Build history of the part. All positions in model axes, mm. Face numbers are marked on the shaded views. A direction names the side the tool comes from. Give positions to 0.01 mm unless a question says otherwise; leave off trailing zeros. Order: outer loops, then holes, each group sorted by start corner. A loop starts at its lowest first (then second) coordinate and runs counter-clockwise, first axis right, second up. Notation, with made-up numbers: (83, 56.5) -> (128, 56.5) arc R30 ccw to (128, 92.5) -> close; hole circle Ø9 at (56, 69.25). An arc over 180 degrees is marked (long way). One line per item, written item: value. Start each with the question number.
(1) Saw through at B-B on y = 10. Count the separate pieces of the cut face and the enclosed holes in it, plus the area to 3 significant figures.
(2) Saw through at A-A on z = -18. Give the cut face in (x, y), plus the area to 3 significant figures.
(3) Saw through at C-C on x = 22.5. Give the cut face in (y, z), plus the area to 3 significant figures.
(4) Pin check, flat tips, straight feed: pin 1 (3.5 mm diameter, centred on x = 7.5, z = 6, fed in from +Y); pin 2 (7.5 mm diameter, centred on y = 16, z = 18, fed in from -X); pin 3 (1 mm diameter, centred on x = -40.5, z = -2.5, fed in from +Y). Stop position of each tip, or through.
(5) Which spindle directions (+Z, -Z, +X, -X, +Y, -Y) get a long thin tool onto all of the face, cutting with end or side? Do the marked faces 1, 2 and 3. Say none if no direction does.
(6) Two-plate mould, pull along Y, no slides. Class the marked faces 4, 5, 6 and 7: +Y half, -Y half, draft (parallel to the pull), parting line (faces both ways), or undercut.
(7) Probe line 1 (X direction, y = 21, z = 13.5); line 2 (X direction, y = 11.5, z = 18); line 3 (X direction, y = 6, z = 25.5). List the from-to ranges inside material, lowest first.
Autodesk Inventor part; units mm, degrees
ref_plane "YZ Plane" through (0, 0, 0) normal (1, 0, 0) x (0, 1, 0)
ref_plane "XZ Plane" through (0, 0, 0) normal (0, 1, 0) x (-1, 0, 0)
ref_plane "XY Plane" through (0, 0, 0) normal (0, 0, 1) x (1, 0, 0)
sketch "Sketch1" plane through (0, 0, 0) normal (0, 1, 0) x (-1, 0, 0)
  line L0 (17.7167, 30.9206) -> (-32.2833, 30.9206)
  line L1 (-32.2833, 30.9206) -> (-32.2833, -19.0794)
  line L2 (-32.2833, -19.0794) -> (17.7167, -19.0794)
  line L3 (17.7167, -19.0794) -> (17.7167, 30.9206)
  line L4 (19.7167, 32.9206) -> (-34.2833, 32.9206)
  line L5 (-34.2833, 32.9206) -> (-34.2833, -21.0794)
  line L6 (-34.2833, -21.0794) -> (19.7167, -21.0794)
  line L7 (19.7167, -21.0794) -> (19.7167, 32.9206)
  line L8 (19.7167, 32.9206) -> (54.7167, 32.9206)
  line L9 (54.7167, 32.9206) -> (54.7167, -21.0794)
  line L10 (54.7167, -21.0794) -> (19.7167, -21.0794)
  line L11 (19.7167, -21.0794) -> (19.7167, 32.9206)
  point P0 (0, 0)
  dimension "d0" = 50
  dimension "d1" = 50
  dimension "d2" = 2
  dimension "d3" = 2
  dimension "d4" = 2
  dimension "d5" = 2
  dimension "d6" = 35
  dimension "d7" = 54
extrude "Extrusion1" add sketch "Sketch1" along normal blind 27 contours L7 L6 L5 L4
sketch "Sketch2" plane through (34.2833, 0, 32.9206) normal (1, 0, 0) x (0, 0, -1)
  line L0 (0, 0) -> (0, 27)
  line L1 (54, 0) -> (54, 27)
  line L2 (0, 0) -> (54, 0)
  line L3 (54, 0) -> (54, 2)
  line L4 (54, 2) -> (0, 2)
  line L5 (0, 2) -> (0, 0)
  point P0 (32.9206, 0)
  dimension "d10" = 2
extrude "Extrusion2" add sketch "Sketch2" against normal blind 89
fillet "Fillet1" radius 2 7 edges at (34.2833, 13.5, 32.9206) (34.2833, 13.5, -21.0794) (-19.7167, 14.5, -21.0794) (-19.7167, 14.5, 32.9206) (34.2833, 0, 5.9206) (-10.2167, 0, 32.9206) (-10.2167, 0, -21.0794)
sketch "Sketch3" plane through (-17.7167, 2, 30.9206) normal (0, 1, 0) x (1, 0, 0)
  line L0 (9, 9) -> (1, 9)
  line L1 (1, 9) -> (1, 17)
  line L2 (1, 17) -> (9, 17)
  line L3 (9, 17) -> (9, 9)
  line L4 (50, 0) -> (0, 0)
  line L5 (0, 0) -> (0, 50)
  line L6 (8.05, 9.95) -> (1.95, 9.95)
  line L7 (1.95, 9.95) -> (1.95, 16.05)
  line L8 (1.95, 16.05) -> (8.05, 16.05)
  line L9 (8.05, 16.05) -> (8.05, 9.95)
  line L10 (0, 25) -> (50, 25)
  line L11 (0, 50) -> (50, 50)
  line L12 (50, 50) -> (50, 0)
  line L13 (9, 41) -> (1, 41)
  line L14 (1, 41) -> (1, 33)
  line L15 (1, 33) -> (9, 33)
  line L16 (9, 33) -> (9, 41)
  line L17 (8.05, 40.05) -> (1.95, 40.05)
  line L18 (1.95, 40.05) -> (1.95, 33.95)
  line L19 (1.95, 33.95) -> (8.05, 33.95)
  line L20 (8.05, 33.95) -> (8.05, 40.05)
  line L21 (36, 25) -> (18, 25)
  line L22 (18, 25) -> (18, 47)
  line L23 (18, 47) -> (36, 47)
  line L24 (36, 47) -> (36, 25)
  line L25 (36, 25) -> (18, 25)
  line L26 (18, 25) -> (18, 15)
  line L27 (18, 15) -> (36, 15)
  line L28 (36, 15) -> (36, 25)
  line L29 (36, 47) -> (18, 47)
  line L30 (18, 47) -> (18, 43)
  line L31 (18, 43) -> (36, 43)
  line L32 (36, 43) -> (36, 47)
  line L33 (36, 15) -> (34, 15)
  line L34 (34, 15) -> (34, 47)
  line L35 (34, 47) -> (36, 47)
  line L36 (36, 47) -> (36, 15)
  line L37 (34, 21) -> (33, 21)
  line L38 (33, 21) -> (33, 22)
  line L39 (33, 22) -> (34, 22)
  line L40 (34, 22) -> (34, 21)
  line L41 (34, 28) -> (33, 28)
  line L42 (33, 28) -> (33, 29)
  line L43 (33, 29) -> (34, 29)
  line L44 (34, 29) -> (34, 28)
  line L45 (34, 39) -> (33, 39)
  line L46 (33, 39) -> (33, 40)
  line L47 (33, 40) -> (34, 40)
  line L48 (34, 40) -> (34, 39)
  point P0 (17.7167, 30.9206)
  dimension "d26" = 9
  dimension "d27" = 8
  dimension "d28" = 1
  dimension "d29" = 6.1
  dimension "d30" = 0.95
  dimension "d31" = 0.95
  dimension "d33" = 25
  dimension "d34" = 25
  dimension "d39" = 16
  dimension "d74" = 22
  dimension "d75" = 18
  dimension "d76" = 18
  dimension "d77" = 10
  dimension "d78" = 18
  dimension "d87" = 4
  dimension "d90" = 2
  dimension "d93" = 6
  dimension "d94" = 1
  dimension "d95" = 1
  dimension "d96" = 3
  dimension "d97" = 3
  dimension "d98" = 1
  dimension "d99" = 1
  dimension "d100" = 10
  dimension "d101" = 1
  dimension "d102" = 1
extrude "Extrusion3" add sketch "Sketch3" along normal blind 15 contours L0 L1 L2 L3
sketch "Sketch4" plane through (-17.7167, 2, 30.9206) normal (0, 1, 0) x (1, 0, 0)
  point P0 (17.7167, 30.9206)
extrude "Extrusion4" add sketch "Sketch3" along normal blind 15 contours L16 L15 L14 L13
fillet "Fillet2" radius 1 8 edges at (-8.7167, 9.5, -2.0794) (-8.7167, 9.5, -10.0794) (-16.7167, 9.5, -2.0794) (-16.7167, 9.5, -10.0794) (-8.7167, 9.5, 13.9206) (-8.7167, 9.5, 21.9206) (-16.7167, 9.5, 21.9206) (-16.7167, 9.5, 13.9206)
sketch "Sketch5" plane through (-17.7167, 27, 30.9206) normal (1, 0, 0) x (0, 0, -1)
  circle A0 centre (25, -11) radius 1.8
  line L0 (50, -25) -> (50, 0)
  line L1 (0, -25) -> (50, -25)
  point P0 (30.9206, -27)
  dimension "d41" = 3.6
  dimension "d42" = 25
  dimension "d43" = 14
extrude "Extrusion5" cut sketch "Sketch5" against normal blind 1
sketch "Sketch6" plane through (-17.7167, 2, 30.9206) normal (0, 1, 0) x (1, 0, 0)
  line L0 (10.5, 9.0139) -> (13.5, 9.0139)
  line L1 (13.5, 9.0139) -> (13.5, 41.0139)
  line L2 (13.5, 41.0139) -> (10.5, 41.0139)
  line L3 (10.5, 41.0139) -> (10.5, 9.0139)
  line L4 (2, 9) -> (8, 9)
  line L5 (8, 41) -> (2, 41)
  line L6 (9, 16) -> (9, 10)
  point P0 (17.7167, 30.9206)
  dimension "d46" = 3
  dimension "d47" = 32
  dimension "d48" = 1.5
extrude "Extrusion6" [suppressed]
sketch "Sketch7" plane through (-4.2167, 2, 21.9067) normal (1, 0, 0) x (0, 0, -1)
  circle A0 centre (15.9861, 14) radius 1.8
  circle A1 centre (15.9861, 14) radius 1.8
  point P0 (21.9067, -2)
  dimension "d51" = 3.6
extrude "Extrusion7" [suppressed]
sketch "Sketch8" plane through (-4.2167, 2, 21.9067) normal (1, 0, 0) x (0, 0, -1)
  line L0 (32.0428, 14) -> (0, 14)
  line L1 (0, 0) -> (0, 14)
  line L2 (0, 14) -> (32, 14)
  line L3 (32, 0) -> (0, 0)
  point P0 (21.9067, -2)
  dimension "d54" = 14
sketch "Sketch9" plane through (-17.7167, 27, 30.9206) normal (1, 0, 0) x (0, 0, -1)
  line L0 (3.6476, -12) -> (44.1553, -12)
  line L1 (44.1553, -12) -> (44.1553, -24)
  line L2 (44.1553, -24) -> (3.6476, -24)
  line L3 (3.6476, -24) -> (3.6476, -12)
  line L4 (0, -25) -> (50, -25)
  point P0 (30.9206, -27)
  dimension "d55" = 12
  dimension "d56" = 1
extrude "Extrusion8" [suppressed]
sketch "Sketch10" plane through (-17.7167, 17, 30.9206) normal (0, 1, 0) x (1, 0, 0)
  line L0 (8.05, 16.05) -> (1.95, 16.05)
  line L1 (2, 17) -> (8, 17)
  line L2 (2.9, 16.05) -> (7.1, 16.05)
  line L3 (7.1, 16.05) -> (7.1, 17)
  line L4 (7.1, 17) -> (2.9, 17)
  line L5 (2.9, 17) -> (2.9, 16.05)
  line L6 (1.95, 9.95) -> (1.95, 16.05)
  line L7 (8.05, 16.05) -> (8.05, 9.95)
  point P0 (17.7167, 30.9206)
  dimension "d59" = 0.95
  dimension "d60" = 0.95
extrude "Extrusion9" cut sketch "Sketch10" against normal blind 10
sketch "Sketch11" plane through (-17.7167, 17, 30.9206) normal (0, 1, 0) x (1, 0, 0)
  line L0 (8, 33) -> (2, 33)
  line L1 (8.05, 33.95) -> (1.95, 33.95)
  line L2 (2.9, 33) -> (7.1, 33)
  line L3 (7.1, 33) -> (7.1, 33.95)
  line L4 (7.1, 33.95) -> (2.9, 33.95)
  line L5 (2.9, 33.95) -> (2.9, 33)
  line L6 (1.95, 33.95) -> (1.95, 40.05)
  line L7 (8.05, 40.05) -> (8.05, 33.95)
  point P0 (17.7167, 30.9206)
  dimension "d63" = 0.95
  dimension "d64" = 0.95
  dimension "d65" = 0.95
extrude "Extrusion10" cut sketch "Sketch11" against normal blind 10
sketch "Sketch12" plane through (-17.7167, 27, 30.9206) normal (1, 0, 0) x (0, 0, -1)
  circle A0 centre (25, -11) radius 3
  circle A1 centre (25, -11) radius 1.8
  point P0 (30.9206, -27)
  dimension "d68" = 6
extrude "Extrusion11" add sketch "Sketch12" along normal blind 2
sketch "Sketch13" plane through (-17.7167, 16, 30.9206) normal (0, 1, 0) x (1, 0, 0)
  line L0 (13.5, 41.0139) -> (13.5, 9.0139)
  line L1 (13.5, 41.0139) -> (10.5, 41.0139)
  line L2 (13.5, 31.0139) -> (10.5, 31.0139)
  line L3 (10.5, 31.0139) -> (10.5, 41.0139)
  line L4 (10.5, 41.0139) -> (13.5, 41.0139)
  line L5 (13.5, 41.0139) -> (13.5, 31.0139)
  line L6 (10.5, 9.0139) -> (13.5, 9.0139)
  point P0 (17.7167, 30.9206)
  dimension "d71" = 10
extrude "Extrusion12" [suppressed]
sketch "Sketch14" plane through (-17.7167, 2, 30.9206) normal (0, 1, 0) x (1, 0, 0)
  point P0 (17.7167, 30.9206)
extrude "Extrusion13" add sketch "Sketch3" along normal blind 9 contours L28 L27 L34 L10 | L10 L34 L31 L24 | L22 L31 L34 L47 L46 L45 L43 L42 L41 L10 | L10 L34 L39 L38 L37 L27 L26 | L31 L34 L23 L24 | L22 L23 L34 L31 | L34 L37 L38 L39 | L41 L42 L43 L34 | L34 L45 L46 L47
sketch "Sketch15" plane through (-17.7167, 11, 30.9206) normal (0, 1, 0) x (1, 0, 0)
  line L0 (36, 47) -> (36, 15)
  line L1 (18, 47) -> (18, 15)
  line L2 (36, 15) -> (18, 15)
  line L3 (18, 15) -> (18, 19)
  line L4 (18, 19) -> (36, 19)
  line L5 (36, 19) -> (36, 15)
  point P0 (17.7167, 30.9206)
  dimension "d81" = 4
extrude "Extrusion14" add sketch "Sketch15" along normal blind 16
extrude "Extrusion16" add sketch "Sketch3" along normal blind 20 contours L31 L34 L23 L24 | L22 L23 L34 L31
extrude "Extrusion17" [suppressed]
extrude "Extrusion18" [suppressed]
extrude "Extrusion19" [suppressed]
extrude "Extrusion20" [suppressed]
sketch "Sketch17" plane through (18.2833, 11, 11.9206) normal (0, 0, -1) x (-1, 0, 0)
  line L0 (0, -9) -> (0, 16)
  line L1 (18, -9) -> (18, 16)
  line L2 (0, 16) -> (18, 16)
  line L3 (18, 16) -> (18, 10)
  line L4 (18, 10) -> (0, 10)
  line L5 (0, 10) -> (0, 16)
  point P0 (18.2833, -11)
  dimension "d109" = 6
extrude "Extrusion21" add sketch "Sketch17" along normal blind 12
sketch "Sketch18" plane through (-17.7167, 11, 30.9206) normal (0, 1, 0) x (1, 0, 0)
  line L0 (18, 19) -> (36, 19)
  line L1 (27, 19) -> (24, 19)
  line L2 (24, 19) -> (24, 23)
  line L3 (24, 23) -> (27, 23)
  line L4 (27, 23) -> (27, 19)
  line L5 (18, 43) -> (18, 19)
  line L6 (24, 27) -> (27, 27)
  line L7 (27, 27) -> (27, 31)
  line L8 (27, 31) -> (24, 31)
  line L9 (24, 31) -> (24, 27)
  line L10 (24, 27) -> (27, 27)
  line L11 (27, 27) -> (27, 23)
  line L12 (27, 23) -> (24, 23)
  line L13 (24, 23) -> (24, 27)
  point P0 (17.7167, 30.9206)
  dimension "d112" = 9
  dimension "d113" = 3
  dimension "d114" = 4
  dimension "d115" = 3
  dimension "d116" = 4
  dimension "d133" = 4
sketch "Sketch19" plane through (-17.7167, 11, 30.9206) normal (0, 1, 0) x (1, 0, 0)
  point P0 (17.7167, 30.9206)
extrude "Extrusion22" add sketch "Sketch18" along normal blind 10 contours L2 L3 L4 L0 | L9 L8 L7 L6
extrude "Extrusion23" add sketch "Sketch18" along normal blind 3 contours L13 L6 L11 L3
sketch "Sketch20" plane through (9.2833, 21, 7.9206) normal (0, 0, -1) x (-1, 0, 0)
  point P0 (9.2833, -21)
sketch "Sketch21" plane through (9.2833, 21, 7.9206) normal (0, 0, -1) x (-1, 0, 0)
  line L0 (0, 0) -> (3, 0)
  line L1 (0, 0) -> (3, 0)
  line L2 (3, 0) -> (3, -3)
  line L3 (3, -3) -> (0, -3)
  line L4 (0, -3) -> (0, 0)
  point P0 (9.2833, -21)
  dimension "d121" = 3
extrude "Extrusion24" add sketch "Sketch21" along normal blind 4
sketch "Sketch22" plane through (18.2833, 2, 15.9206) normal (1, 0, 0) x (0, 0, -1)
  line L0 (5.5, 7) -> (26.5, 7)
  line L1 (26.5, 7) -> (26.5, 0)
  line L2 (26.5, 0) -> (5.5, 0)
  line L3 (5.5, 0) -> (5.5, 7)
  line L4 (4, 9) -> (28, 9)
  line L5 (28, 9) -> (28, 20)
  point P0 (15.9206, -2)
  dimension "d124" = 2
  dimension "d125" = 7
  dimension "d126" = 21
  dimension "d129" = 1.5
extrude "Extrusion25" cut sketch "Sketch22" against normal blind 20
sketch "Sketch23" plane through (18.2833, 11, -0.0794) normal (0, 0, -1) x (-1, 0, 0)
  line L0 (18, 16) -> (0, 16)
  line L1 (0, 16) -> (0, 10)
  line L2 (18, 16) -> (0, 16)
  line L3 (0, 16) -> (0, 13)
  line L4 (0, 13) -> (18, 13)
  line L5 (18, 13) -> (18, 16)
  point P0 (18.2833, -11)
  dimension "d130" = 3
extrude "Extrusion26" cut sketch "Sketch23" against normal blind 10
equation "\"d1\" = d0"
equation "\"d76\" = d75"
equation "\"d98\" = d95"
equation "\"d99\" = d94"
equation "\"d101\" = d99"
equation "\"d102\" = d95"
equation "\"d54\" = d43"
equation "\"d115\" = d113"
equation "\"d116\" = d114"
properties part number "ohisje"
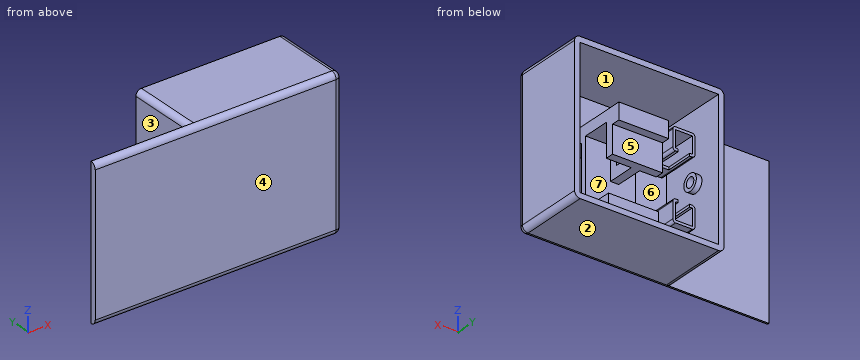
Results below:
1. separate pieces: 4
1. enclosed holes: 1
1. area: 1,030 mm²
2. outline: (-54.72, 0) -> (32.28, 0) arc R2 ccw to (34.28, 2) -> (34.28, 27) -> (32.28, 27) -> (32.28, 2) -> (-17.72, 2) -> (-17.72, 27) -> (-19.72, 27) -> (-19.72, 2) -> (-54.72, 2) -> close
2. area: 277 mm²
3. outline: (0, -19.08) arc R2 ccw to (2, -21.08) -> (27, -21.08) -> (27, -19.08) -> (2, -19.08) -> (2, 30.92) -> (27, 30.92) -> (27, 32.92) -> (2, 32.92) arc R2 ccw to (0, 30.92) -> close
3. area: 206 mm²
4. pin 1: stops at y = 24
4. pin 2: stops at x = -19.72
4. pin 3: stops at y = 2
5. face 1: +Y
5. face 2: -Z, +X, -X, +Y, -Y
5. face 3: +Z, -Z, -X, +Y
6. face 4: -Y half
6. face 5: +Y half
6. face 6: undercut
6. face 7: undercut
7. line 1: x = -19.72 to -17.72, 0.28 to 18.28, 32.28 to 34.28
7. line 2: x = -19.72 to -17.72, -16.72 to -15.77, -9.67 to -8.72, 32.28 to 34.28
7. line 3: x = -19.72 to -17.72, 32.28 to 34.28
